from build123d import *

# Parameters (mm, degrees)
F0_W      = 300
F0_H      = 200
F1_DEPTH  = 300
F2_W      = 260
F2_H      = 260
F3_DEPTH  = 421.64
F4_SIZE   = 10
F5_R      = 10
F6_SIZE   = 10
F7_R      = 8.75
F8_DEPTH  = 79.502
F7_R_2    = 15.75
F9_DEPTH  = 20
F10_R     = 99.99999
F11_R     = 50
F12_DEPTH = 145.034
F13_D     = 12.1
F14_SIZE  = 5
F16_DEPTH = 25
F20_D     = 15.5
F20_DEPTH = 44.0944
F20_START = 0.8055971
F20_TIP   = 4.6566697975


# Not quite as in the source:
# - a fillet or chamfer is up to 0.001 mm smaller than in the source, because OpenCascade refuses the exact size


with BuildPart() as f1:
    # F0 (on Top) → F1 (new body)
    with BuildSketch(Plane.XY):
        Rectangle(F0_W, F0_H)
    extrude(amount=F1_DEPTH)

    # F2 (on face) → F3 (cut)
    with BuildSketch(Plane.XZ.offset(100)):
        with Locations((20, 170)):
            Rectangle(F2_W, F2_H)
    extrude(amount=-F3_DEPTH, mode=Mode.SUBTRACT)

    # F4
    f4_edges = [f1.edges().sort_by_distance(p)[0] for p in [
        (150, -100, 20),
        (150, 100, 20),
    ]]
    chamfer(f4_edges, length=F4_SIZE)

    # F5
    f5_edges = [f1.edges().sort_by_distance(p)[0] for p in [
        (-110, 0, 40),
    ]]
    fillet(f5_edges, radius=F5_R)

    # F6
    f6_edges = [f1.edges().sort_by_distance(p)[0] for p in [
        (-150, 0, 0),
    ]]
    chamfer(f6_edges, length=F6_SIZE)

    # F7 (on face) → F8 (cut)
    with BuildSketch(Plane.XY.offset(40)):
        with Locations((110, -60)):
            Circle(F7_R)
        with Locations((110, 60)):
            Circle(F7_R)
        with Locations((-10, 60)):
            Circle(F7_R)
        with Locations((-10, -60)):
            Circle(F7_R)
    extrude(amount=-F8_DEPTH, mode=Mode.SUBTRACT)

    # F7 (on face) → F9 (cut)
    with BuildSketch(Plane.XY.offset(40)):
        with Locations((-10, 60)):
            Circle(F7_R_2)
        with Locations((-10, 60)):
            Circle(F7_R, mode=Mode.SUBTRACT)
        with Locations((-10, -60)):
            Circle(F7_R_2)
        with Locations((-10, -60)):
            Circle(F7_R, mode=Mode.SUBTRACT)
        with Locations((110, -60)):
            Circle(F7_R_2)
        with Locations((110, -60)):
            Circle(F7_R, mode=Mode.SUBTRACT)
        with Locations((110, 60)):
            Circle(F7_R_2)
        with Locations((110, 60)):
            Circle(F7_R, mode=Mode.SUBTRACT)
    extrude(amount=-F9_DEPTH, mode=Mode.SUBTRACT)

    # F10 (radius 100 in the source; OpenCascade refuses exactly that, so slightly less here)
    f10_edges = [f1.edges().sort_by_distance(p)[0] for p in [
        (-130, -100, 300),
        (-130, 100, 300),
    ]]
    fillet(f10_edges, radius=F10_R)

    # F11 (on face) → F12 (cut)
    with BuildSketch(Plane.YZ.offset(-110)):
        with Locations((0, 210.0496292114)):
            Circle(F11_R)
    extrude(amount=-F12_DEPTH, mode=Mode.SUBTRACT)

    # F13 (through all)
    with Locations(Plane.YZ.offset(-110)):
        with Locations((-72, 210.0496292114), (0, 282.0496292114), (71.9983499009, 210.5370833633), (0, 138.0496292114)):
            Hole(F13_D / 2)

    # F14
    f14_edges = [f1.edges().sort_by_distance(p)[0] for p in [
        (-150, -50, 210.049629),
        (-110, -50, 210.049629),
    ]]
    chamfer(f14_edges, length=F14_SIZE)

    # F15 (on Front) → F16 (join, symmetric)
    with BuildSketch(Plane.XZ):
        Polygon((-51.5841689292, 39.5744924862), (-111.5841689292, 99.5744924862), (-111.5841689292, 39.5744924862), align=None)
    extrude(amount=F16_DEPTH, both=True)

    # F20
    # its depths count from where the whole tool has entered the part; down to there all is cleared
    with Locations(Plane(origin=(0, -166.0770217272, 185.5655664485), x_dir=(1, 0, 0), z_dir=(0, -0.6668944822, 0.7451521654)).offset(-F20_START)):
        with Locations((-129.2792707682, 138.2966190577)):
            Hole(F20_D / 2, depth=F20_DEPTH)
            with Locations((0, 0, -(F20_DEPTH + F20_TIP / 2))):  # 118° drill point
                Cone(0, F20_D / 2, F20_TIP, mode=Mode.SUBTRACT)


solid = f1.part
Geometry: final body of the model. Coordinates: model frame, mm. A direction names the side the tool comes from. Round coordinates to 2 decimals unless told otherwise and drop trailing zeros. Order: outer loops, then holes, each group sorted by start corner. A loop starts at its lowest first (then second) coordinate and runs counter-clockwise, first axis right, second up. Notation, with made-up numbers: (-20.75, 49) -> (9.25, 49) arc R22 cw to (9.25, 67) -> close; hole circle Ø9 at (47.5, -10). An arc over 180 degrees is marked (long way). Put each result on its own line as item: value. Start each with the question number.
Q1. Reachability of faces 4 (the cylindrical face through (125.023, 64.731, 30.14)), 5 (the cylindrical face through (-106.99, -61.98, 42.85)), 6 (the cylindrical face through (-130.28, 66.41, 208.22)) from +Z, -Z, +X, -X, +Y, -Y: full face, straight path, thin tool, end or side. Return the list, or none.
Q2. Section C-C on z = 24.5. Return the cut outline in (x, y).
Q3. Section B-B on x = -10. Return the cut outline in (y, z).
Q4. Section D-D on x = -129. Give the number of separate pieces and of enclosed holes in the cut face, and give its area (3 significant figures).
Q5. Pull-direction query (Z, two-part tool) for faces 1 (the cylindrical face through (-106.99, 63.03, 42.85)), 2 (the cylindrical face through (-129.79, 23.07, 165.69)), 3 (the cylindrical face through (101.26, -59.62, 10.14)); classes: +Z half, -Z half, draft (parallel to the pull), parting line (faces both ways), or undercut.
Q6. Line query: probe 1 along Y at (x, z) = (-10, 24); probe 2 along X at (y, z) = (-40, 63); probe 3 along Z at (x, y) = (93, -63). Output: solid intervals per line, ascending.
Q7. Section A-A on y = 60. Return the cut outline in (x, z), and give its area (3 significant figures).
Q8. First-contact query: pin 1 (19 mm diameter, centred on x = -10, y = 60, fed in from +Z); pin 2 (12 mm diameter, centred on x = -20.5, y = 57, fed in from +Z); pin 3 (16 mm diameter, centred on x = 110, y = -60, fed in from +Z); pin 4 (25 mm diameter, centred on x = 110, y = -60, fed in from -Z). Flat tips, straight axial feed; report the tip coordinate or a pass-through.
Ans:
1. face 4: +Z
1. face 5: +Z, +X, -Y
1. face 6: +X, -X
2. outline: (-150, -100) -> (140, -100) -> (150, -90) -> (150, 90) -> (140, 100) -> (-150, 100) -> close; hole circle Ø31.5 at (-10, -60); hole circle Ø31.5 at (-10, 60); hole circle Ø31.5 at (110, -60); hole circle Ø31.5 at (110, 60)
3. outline: (-100, 0) -> (-68.75, 0) -> (-68.75, 20) -> (-75.75, 20) -> (-75.75, 40) -> (-100, 40) -> close; (-51.25, 0) -> (51.25, 0) -> (51.25, 20) -> (44.25, 20) -> (44.25, 40) -> (-44.25, 40) -> (-44.25, 20) -> (-51.25, 20) -> close; (68.75, 0) -> (100, 0) -> (100, 40) -> (75.75, 40) -> (75.75, 20) -> (68.75, 20) -> close
4. separate pieces: 1
4. enclosed holes: 4
4. area: 46,700 mm2
5. face 1: +Z half
5. face 2: undercut
5. face 3: draft
6. probe 1: y = -100 to -75.75, -44.25 to 44.25, 75.75 to 100
6. probe 2: x = -150 to -110
6. probe 3: z = 0 to 40
7. outline: (-150, 10) -> (-140, 0) -> (-18.75, 0) -> (-18.75, 20) -> (-25.75, 20) -> (-25.75, 40) -> (-100, 40) arc R10 cw to (-110, 50) -> (-110, 280) -> (-150, 280) -> close; (-1.25, 0) -> (101.25, 0) -> (101.25, 20) -> (94.25, 20) -> (94.25, 40) -> (5.75, 40) -> (5.75, 20) -> (-1.25, 20) -> close; (118.75, 0) -> (150, 0) -> (150, 40) -> (125.75, 40) -> (125.75, 20) -> (118.75, 20) -> close
7. area: 19,600 mm2
8. pin 1: stops at z = 20
8. pin 2: stops at z = 40
8. pin 3: passes through
8. pin 4: stops at z = 0
